Input: part model. Units: mm. Frame: model coordinates. Face numbers are marked on the shaded views. Coordinates: 2 decimals unless noted, no trailing zeros. Write each loop counter-clockwise with the first axis right and the second up, starting at its lowest first coordinate (ties: lowest second). Pieces come first, ordered by that corner, then holes.
1) Section query B-B (z = 2.75). Output: boundary loops of the cut face in (x, y), then the cut area to 3 significant figures.
2) Line query: L1, parallel to Y at x = 0, z = 2.75; L2, parallel to Y at x = -0.75, z = 1.05; L3, parallel to Z at x = 0, y = -0.5. Output: solid intervals per line, ascending.
3) Section query A-A (z = 4.2). Output: boundary loops of the cut face in (x, y).
4) Draft query along X for the marked faces 1, 2 and 3. Return one class per face: pulls with the +X half, pulls with the -X half, needs draft (parallel to the pull), parting line crosses it, or undercut.
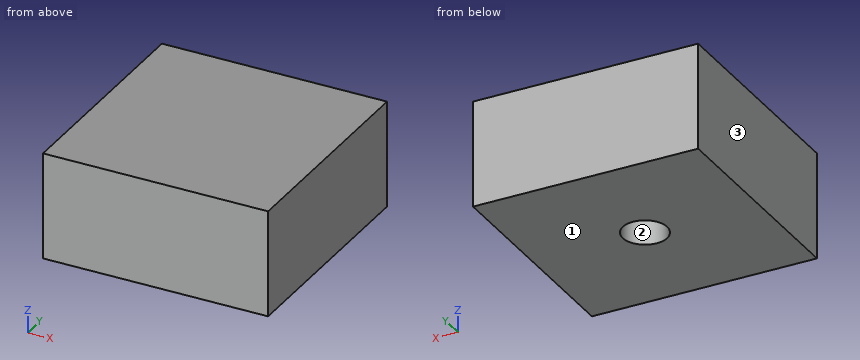
from build123d import *

# Parameters (mm, degrees)
SKETCH1_W                       = 12.7
SKETCH1_H                       = 12.7
BOSS_EXTRUDE1_DEPTH             = 6
TAP_DRILL_FOR_M3X0_5_TAP3_D     = 2.5
TAP_DRILL_FOR_M3X0_5_TAP3_DEPTH = 4
TAP_DRILL_FOR_M3X0_5_TAP3_TIP   = 0.751075774


with BuildPart() as part:
    # Sketch1 → Boss-Extrude1 (new body)
    with BuildSketch(Plane.XY):
        Rectangle(SKETCH1_W, SKETCH1_H)
    extrude(amount=BOSS_EXTRUDE1_DEPTH)

    # Tap Drill for M3x0.5 Tap3
    with Locations(Plane(origin=(0, 0, 0), x_dir=(1, 0, 0), z_dir=(0, 0, -1))):
        with Locations((0, 0)):
            Hole(TAP_DRILL_FOR_M3X0_5_TAP3_D / 2, depth=TAP_DRILL_FOR_M3X0_5_TAP3_DEPTH)
            with Locations((0, 0, -(TAP_DRILL_FOR_M3X0_5_TAP3_DEPTH + TAP_DRILL_FOR_M3X0_5_TAP3_TIP / 2))):  # 118° drill point
                Cone(0, TAP_DRILL_FOR_M3X0_5_TAP3_D / 2, TAP_DRILL_FOR_M3X0_5_TAP3_TIP, mode=Mode.SUBTRACT)


solid = part.part
Answer:
1. outline: (-6.35, -6.35) - (6.35, -6.35) - (6.35, 6.35) - (-6.35, 6.35) - close; hole circle Ø2.5 at (0, 0)
1. area: 156 mm2
2. L1: y = -6.35 to -1.25, 1.25 to 6.35
2. L2: y = -6.35 to -1, 1 to 6.35
2. L3: z = 4.45 to 6
3. outline: (-6.35, -6.35) - (6.35, -6.35) - (6.35, 6.35) - (-6.35, 6.35) - close; hole circle Ø1.83 at (0, 0)
4. face 1: needs draft
4. face 2: undercut
4. face 3: pulls with the -X half
